For this review, take the finished solid that the model builds, in its own axes (mm). A direction names the side the tool comes from. Coordinates: 2 decimals unless noted, no trailing zeros. Write each loop counter-clockwise with the first axis right and the second up, starting at its lowest first coordinate (ties: lowest second). Pieces come first, ordered by that corner, then holes.
```python
from build123d import *

# Parameters (mm, degrees)
SKETCH_1_R      = 2
SKETCH_1_R_2    = 1.8
SKETCH_1_R_3    = 23.45
EXTRUDE_1_DEPTH = 1.09
EXTRUDE_START   = -20.5
SKETCH_2_R      = 24.5
SKETCH_2_R_2    = 23.45
EXTRUDE_2_DEPTH = 20.5
FILLET_1_R      = 2
SKETCH_3_R      = 1.5
EXTRUDE_3_DEPTH = 11.5


with BuildPart() as part:
    # Эскиз1 → Бобышка-Вытянуть1 (new body)
    with BuildSketch(Plane.XY):
        Polygon((-30.964466094, 34.5), (-34.5, 30.964466094), (-34.5, 20.464466094), (-36, 18.956328052), (-36, 16.901005102), (-32.3, 16.901005102), (-32.3, 14.901005102), (-36, 14.901005102), (-36, -14.901005102), (-32.3, -14.901005102), (-32.3, -16.901005102), (-36, -16.901005102), (-36, -18.956328052), (-34.5, -20.464466094), (-34.5, -30.964466094), (-30.964466094, -34.5), (-20.464466094, -34.5), (-18.956328052, -36), (-16.901005102, -36), (-16.901005102, -32.3), (-14.901005102, -32.3), (-14.901005102, -36), (14.901005102, -36), (14.901005102, -32.3), (16.901005102, -32.3), (16.901005102, -36), (18.956328052, -36), (20.464466094, -34.5), (30.964466094, -34.5), (34.5, -30.964466094), (34.5, -20.464466094), (36, -18.956328052), (36, -16.901005102), (32.3, -16.901005102), (32.3, -14.901005102), (36, -14.901005102), (36, 14.901005102), (32.3, 14.901005102), (32.3, 16.901005102), (36, 16.901005102), (36, 18.956328052), (34.5, 20.464466094), (34.5, 30.964466094), (30.964466094, 34.5), (20.464466094, 34.5), (18.956328052, 36), (16.901005102, 36), (16.901005102, 32.3), (14.901005102, 32.3), (14.901005102, 36), (-14.901005102, 36), (-14.901005102, 32.3), (-16.901005102, 32.3), (-16.901005102, 36), (-18.956328052, 36), (-20.464466094, 34.5), align=None)
        with Locations((-30, 30)):
            Circle(SKETCH_1_R, mode=Mode.SUBTRACT)
        with Locations((-30, 0)):
            Circle(SKETCH_1_R_2, mode=Mode.SUBTRACT)
        with Locations((30, 30)):
            Circle(SKETCH_1_R, mode=Mode.SUBTRACT)
        with Locations((0, 30)):
            Circle(SKETCH_1_R_2, mode=Mode.SUBTRACT)
        with Locations((30, -30)):
            Circle(SKETCH_1_R, mode=Mode.SUBTRACT)
        with Locations((30, 0)):
            Circle(SKETCH_1_R_2, mode=Mode.SUBTRACT)
        with Locations((-30, -30)):
            Circle(SKETCH_1_R, mode=Mode.SUBTRACT)
        with Locations((0, -30)):
            Circle(SKETCH_1_R_2, mode=Mode.SUBTRACT)
        Circle(SKETCH_1_R_3, mode=Mode.SUBTRACT)
    extrude(amount=EXTRUDE_1_DEPTH)

    # Эскиз2 → Бобышка-Вытянуть2 (add)
    with BuildSketch(Plane.XY.offset(1.09).offset(EXTRUDE_START)):
        Circle(SKETCH_2_R)
        Circle(SKETCH_2_R_2, mode=Mode.SUBTRACT)
    extrude(amount=EXTRUDE_2_DEPTH)

    # Скругление1
    fillet_1_edges = [part.edges().sort_by_distance(p)[0] for p in [
        (-23.45, 0, 1.09),
        (-24.5, 0, 0),
    ]]
    fillet(fillet_1_edges, radius=FILLET_1_R)

    # Эскиз3 → Бобышка-Вытянуть3 (add)
    with BuildSketch(Plane(origin=(0, 0, -19.41), x_dir=(-1, 0, 0), z_dir=(0, 0, -1))):
        with BuildLine():
            Line((-18, -19.125), (-18, 19.125))
            ThreePointArc((-18, 19.125), (-16.828427125, 21.953427125), (-14, 23.125))
            Line((-14, 23.125), (9.094464209, 23.125))
            ThreePointArc((9.094464209, 23.125), (11.445269302, 22.361312008), (12.898433585, 20.361857708))
            Line((12.898433585, 20.361857708), (17.803969376, 5.274828861))
            ThreePointArc((17.803969376, 5.274828861), (17.95068839, 4.664119098), (18, 4.037971153))
            Line((18, 4.037971153), (18, -4.037971153))
            ThreePointArc((18, -4.037971153), (17.95068839, -4.664119098), (17.803969376, -5.274828861))
            Line((17.803969376, -5.274828861), (12.898433585, -20.361857708))
            ThreePointArc((12.898433585, -20.361857708), (11.445269302, -22.361312008), (9.094464209, -23.125))
            Line((9.094464209, -23.125), (-14, -23.125))
            ThreePointArc((-14, -23.125), (-16.828427125, -21.953427125), (-18, -19.125))
        make_face()
        Circle(SKETCH_3_R, mode=Mode.SUBTRACT)
    extrude(amount=EXTRUDE_3_DEPTH)


solid = part.part
```
Q1. Add section D-D (z = -23.5). State the section outline as (x, y) points (3 decimals), then the cut area to 3 significant figures.
Ans:
outline: (-18, -4.038) arc R4 ccw to (-17.804, -5.275) - (-12.898, -20.362) arc R4 ccw to (-9.094, -23.125) - (14, -23.125) arc R4 ccw to (18, -19.125) - (18, 19.125) arc R4 ccw to (14, 23.125) - (-9.094, 23.125) arc R4 ccw to (-12.898, 20.362) - (-17.804, 5.275) arc R4 ccw to (-18, 4.038) - close; hole circle Ø3 at (0, 0)
area: 1,540 mm2
Q2. Clearance check with flat-ended pins moving along their axes: pin 1 Ø1.5 at (x, z) = (21.5, -18.5) entering from -Y; pin 2 Ø0.9 at (y, z) = (33.5, 0.5) entering from +X; pin 3 Ø1.2 at (y, z) = (-33.5, 1) entering from +X. State where each tip first meets the part, or that it passes through.
Ans:
pin 1: stops at y = -13.03
pin 2: stops at x = 32.41
pin 3: stops at x = 32.56
Q3. Draft analysis for pull direction Z (two halves, no side actions). For faces 6 (the cylindrical face through (16.8, -21.98, -25.08)), 7 (the flat face through (-10.7, 22.4, -19.41)), 8 (the flat face through (-25, 9, 1.09)), 9 (the flat face through (-10.54, -22.29, -19.41)), state which applies: +Z half, -Z half, draft (parallel to the pull), parting line (faces both ways), or undercut.
Ans:
face 6: draft
face 7: undercut
face 8: +Z half
face 9: undercut
Q4. Add section C-C (y = -30). State the section outline as (x, z) points.
Ans:
outline: (-34.5, 0) - (-32, 0) - (-32, 1.09) - (-34.5, 1.09) - close; (-28, 0) - (-1.8, 0) - (-1.8, 1.09) - (-28, 1.09) - close; (1.8, 0) - (28, 0) - (28, 1.09) - (1.8, 1.09) - close; (32, 0) - (34.5, 0) - (34.5, 1.09) - (32, 1.09) - close
Q5. Add section A-A (y = 0). Give the number of separate pieces and of enclosed holes in the cut face, then the cut area to 3 significant figures.
Ans:
separate pieces: 6
enclosed holes: 0
area: 440 mm2
Q6. Tool access review of faces 1 (the flat face through (4, 0, -19.41)), 2 (the flat face through (3, 23.125, -25)), 3 (the flat face through (2, -23.125, -25)), 4 (the flat face through (15, 21, -19.41)), 5 (the flat face through (24, 0, -19.41)): name each direction out of +Z, -Z, +X, -X, +Y, -Y from which nothing blocks a thin tool from reaching the whole face with its end or side.
Ans:
face 1: +Z
face 2: -Z, +X, -X, +Y
face 3: -Z, +X, -X, -Y
face 4: +X, +Y
face 5: -Z, +X, +Y, -Y
Q7. For probe 1 along Y at (x, z) = (0, -6); probe 2 along Z at (x, y) = (20.5, -32); probe 3 along Z at (x, y) = (-6.5, 3), list the stretches that pass through material, from the lowest coordinate up.
Ans:
probe 1: y = -24.5 to -23.45, 23.45 to 24.5
probe 2: z = 0 to 1.09
probe 3: z = -30.91 to -19.41
